from build123d import *

# Parameters (mm, degrees)
ESQUISSE1_W                             = 14.2
ESQUISSE1_H                             = 14.4
ENL_VEMENT_DE_MATI_RE_R_VOLUTION2_ANGLE = 180
ENL_V_MAT_EXTRU_1_REACH                 = 26.827
ENL_V_MAT_EXTRU_1_END_RADIUS            = 12.7
ESQUISSE5_R                             = 7
DIAM_TRE_DU_PER_AGE_2_5_2_5_1_D         = 2.5


with BuildPart() as part:
    # Esquisse1 → Révolution1 (revolve)
    with BuildSketch(Plane.XY):
        with Locations((7.1, 7.2)):
            Rectangle(ESQUISSE1_W, ESQUISSE1_H)
    revolve(axis=Axis((14.2, 0, 0), (-1, 0, 0)))

    # Esquisse4 → Enlèvement de matière-Révolution2 (revolve, cut)
    with BuildSketch(Plane(origin=(14.2, 0, 0), x_dir=(0, 0, -1), z_dir=(1, 0, 0))):
        with BuildLine():
            Line((5.69655858, -11.350736555), (-5.69655858, 11.350736555))
            Line((-5.69655858, 11.350736555), (-5.698821877, 11.349600399))
            ThreePointArc((-5.698821877, 11.349600399), (-11.350168533, -5.697690257), (5.69655858, -11.350736555))
        make_face()
    revolve(axis=Axis((14.2, -12.018635625, -6.031754993), (0, -0.8937587838633266, -0.4485479196999441)), revolution_arc=ENL_VEMENT_DE_MATI_RE_R_VOLUTION2_ANGLE, mode=Mode.SUBTRACT)

    # Enlèv. mat.-Extru.1: up to this sphere (the profile starts outside it)
    enl_v_mat_extru_1_end = Location((14.2, 0, 0)) * Sphere(ENL_V_MAT_EXTRU_1_END_RADIUS, mode=Mode.PRIVATE)
    # Esquisse5 → Enlèv. mat.-Extru.1 (cut, up to the surface)
    with BuildSketch(Plane.ZY, mode=Mode.PRIVATE) as enl_v_mat_extru_1_sk1:
        with Locations(Location((0, 0, 0), (0, 0, 270))):
            Circle(ESQUISSE5_R)
    enl_v_mat_extru_1_tool1 = extrude(enl_v_mat_extru_1_sk1.sketch, amount=-ENL_V_MAT_EXTRU_1_REACH, mode=Mode.PRIVATE) - enl_v_mat_extru_1_end
    add(enl_v_mat_extru_1_tool1.solids().sort_by_distance((0, 0, 0))[0], mode=Mode.SUBTRACT)

    # Diamètre du perçage Ø2.5 (2.5)1 (through all)
    with Locations(Plane.ZY):
        with Locations((-10.672597122, -0.765291239), (5.999060215, -8.860094612), (4.673536907, 9.625385851)):
            Hole(DIAM_TRE_DU_PER_AGE_2_5_2_5_1_D / 2)


solid = part.part
Can you work these out from the model? Positions are in its coordinate system, mm. Round coordinates to 2 decimals unless told otherwise and drop trailing zeros. Loops run counter-clockwise (first coordinate to the right, second up) from the corner with the lowest first, then second, coordinate; pieces in that order, holes last. Notation, with made-up numbers: (25, 34.25) - (44, 34.25) arc R30 cw to (44, 66.25) - close; hole circle Ø2 at (47.25, -32.5). An arc over 180 degrees is marked (long way). Write item = value, one per line. Start each with the question number.
(1) If we section it at D-D (x = 9.25): Please give me the cut outline in (y, z).
(2) If we section it at C-C (y = 3): Please give me the cut outline in (x, z).
(3) If I drill on probe 1 along Z at (x, y) = (11.5, -3.25); probe 2 along Y at (x, z) = (2.25, -10.25); probe 3 along Y at (x, z) = (6.25, 6.25), over which ranges is the centre line in solid material (lowest first)? Write a range as [from, to].
(4) If we section it at B-B (y = 0): Please give me the cut outline in (x, z), and give its area (3 significant figures).
(5) For P1, Ø4, axis at x = 9.5, y = 7.5, coming from the -Z side; P2, Ø2, axis at y = -1, z = 6, coming from the +X side; P3, Ø6, axis at x = 6, z = -4.5, coming from the +Y side, each with a flat end and sliding along its axis, tell me the tip position at first contact or that it passes through.
(6) If we section it at A-A (z = 0): Please give me the cut outline in (x, y).
(7) If we mould it in two halves opening along Y, with no side actions, what happens to faces 1 (the face through (1.776, -6.466, -2.681)), 2 (the face through (0, 7, 3)), 3 (the face through (7.199, 13.735, -4.325))? For each: released by +Y, released by -Y, zero draft, split by the parting line, or undercut.
Ans:
q1.outline = circle Ø28.8 at (0, 0); hole (-10.11, 5.89) arc R11.7 ccw to (-1.62, -11.58) arc R1.25 ccw to (-0.05, -11.7) arc R11.7 ccw to (10.84, 4.39) arc R1.25 ccw to (10.15, 5.81) arc R11.7 ccw to (-9.22, 7.2) arc R1.25 ccw to start
q2.outline = (0, -14.08) - (14.2, -14.08) - (14.2, -12.34) arc R12.34 cw to (3.6, -6.32) - (0, -6.32) - close; (0, 6.32) - (3.6, 6.32) arc R12.34 cw to (14.2, 12.34) - (14.2, 14.08) - (0, 14.08) - close
q3.probe_1 = [-14.03, -11.98], [11.98, 14.03]
q3.probe_2 = [-10.11, -1.94], [0.41, 10.11]
q3.probe_3 = [-12.97, -10.08], [7.68, 12.97]
q4.outline = (0, -14.4) - (14.2, -14.4) - (14.2, -12.7) arc R12.7 cw to (9.17, -11.66) - (0, -11.66) - close; (0, -9.68) - (5.98, -9.68) arc R12.7 cw to (3.6, -7) - (0, -7) - close; (0, 7) - (3.6, 7) arc R12.7 cw to (14.2, 12.7) - (14.2, 14.4) - (0, 14.4) - close
q4.area = 111 mm²
q5.P1 = -13.31
q5.P2 = 3.66
q5.P3 = 14.32
q6.outline = (0, -14.4) - (14.2, -14.4) - (14.2, -12.7) arc R12.7 cw to (3.6, -7) - (0, -7) - close; (0, 7) - (3.6, 7) arc R12.7 cw to (14.2, 12.7) - (14.2, 14.4) - (0, 14.4) - close
q7.face_1 = undercut
q7.face_2 = zero draft
q7.face_3 = split by the parting line
